Build history of the part. All positions in model axes, mm. A direction names the side the tool comes from. Coordinates: 2 decimals unless noted, no trailing zeros. Loops run counter-clockwise (first coordinate to the right, second up) from the corner with the lowest first, then second, coordinate; pieces in that order, holes last. Notation, with made-up numbers: (18, 10.25) -> (63, 10.25) arc R26 cw to (63, 40.25) -> close; hole circle Ø4 at (64, 55.5). An arc over 180 degrees is marked (long way). One line per item, written item: value. Start each with the question number.
```python
from build123d import *

# Parameters (mm, degrees)
SKETCH2_W           = 111
SKETCH2_H           = 19.962120642
SKETCH2_R           = 5.135
SKETCH2_W_2         = 26.757359312
SKETCH2_H_2         = 45.518939679
BOSS_EXTRUDE1_DEPTH = 15


with BuildPart() as part:
    # Sketch2 → Boss-Extrude1 (new body)
    # profile 1 of 2: a face of its own
    with BuildSketch(Plane(origin=(0, 0, 0), x_dir=(1, 0, 0), z_dir=(0, 1, 0))):
        Rectangle(SKETCH2_W, SKETCH2_H)
        with Locations(Location((0, 0, 0), (0, 0, 270))):
            Circle(SKETCH2_R, mode=Mode.SUBTRACT)
    # profile 2 of 2: a face of its own
    with BuildSketch(Plane(origin=(0, 0, 0), x_dir=(1, 0, 0), z_dir=(0, 1, 0))):
        with Locations((0, -32.740530161)):
            Rectangle(SKETCH2_W_2, SKETCH2_H_2)
    extrude(amount=BOSS_EXTRUDE1_DEPTH)


solid = part.part
```
Item 1: Band-saw the part on D-D, the plane x = -19. List the corners of the cut face in (y, z), and give its area (3 significant figures).
Item 2: Drop flat-ended pins along their axis: pin 1 Ø8 at (x, y) = (-23.5, 11) entering from +Z; pin 2 Ø6 at (y, z) = (8.5, 19.5) entering from -X; pin 3 Ø4.5 at (y, z) = (5, 34.5) entering from +X. Give the stop position or say it passes through.
Item 3: Two-plate mould, pull along Z, no slides. Class faces 4 (the face through (55.5, 7, 0)), 5 (the face through (0, 7, 55.5)), 6 (the face through (1.54, 7.4, 4.9)): +Z half, -Z half, draft (parallel to the pull), parting line (faces both ways), or undercut.
Item 4: Probe probe 1 along X at (y, z) = (7.5, 0) (3 decimals); probe 2 along Z at (x, y) = (-35.5, 6.75); probe 3 along X at (y, z) = (10.75, 39). List the from-to ranges inside material, lowest first.
Item 5: Band-saw the part on A-A, the plane x = 0. List the corners of the cut face in (y, z) (3 decimals), and give its area (3 significant figures).
Item 6: Tool access for faces 1 (the face through (-1, 15, 15)), 2 (the face through (13.379, 7, 33)), 3 (the face through (-35, 7, 9.981)): list every direction of +Z, -Z, +X, -X, +Y, -Y with a clear straight run to the whole face (end or side of a thin tool).
Item 7: Band-saw the part on B-B, the plane z = 0. List the corners of the cut face in (x, y) (3 decimals), and give its area (3 significant figures).
Item 8: Band-saw the part on C-C, the plane y = 5. List the corners of the cut face in (x, z) (3 decimals), and give its area (3 significant figures).
Worked out:
1. outline: (0, -9.98) -> (15, -9.98) -> (15, 9.98) -> (0, 9.98) -> close
1. area: 299 mm²
2. pin 1: stops at z = 9.98
2. pin 2: stops at x = -13.38
2. pin 3: stops at x = 13.38
3. face 4: draft
3. face 5: +Z half
3. face 6: undercut
4. probe 1: x = -55.5 to -5.135, 5.135 to 55.5
4. probe 2: z = -9.98 to 9.98
4. probe 3: x = -13.38 to 13.38
5. outline: (0, -9.981) -> (15, -9.981) -> (15, -5.135) -> (0, -5.135) -> close; (0, 5.135) -> (15, 5.135) -> (15, 55.5) -> (0, 55.5) -> close
5. area: 828 mm²
6. face 1: +Z, -Z, +X, -X, +Y
6. face 2: +Z, +X, +Y, -Y
6. face 3: +Z, -X, +Y, -Y
7. outline: (-55.5, 0) -> (-5.135, 0) -> (-5.135, 15) -> (-55.5, 15) -> close; (5.135, 0) -> (55.5, 0) -> (55.5, 15) -> (5.135, 15) -> close
7. area: 1,510 mm²
8. outline: (-55.5, -9.981) -> (55.5, -9.981) -> (55.5, 9.981) -> (13.379, 9.981) -> (13.379, 55.5) -> (-13.379, 55.5) -> (-13.379, 9.981) -> (-55.5, 9.981) -> close; hole circle Ø10.27 at (0, 0)
8. area: 3,350 mm²
